Read the model definition and answer for the solid it produces. Units are mm, in the model's axes. Give positions to 0.01 mm unless a question says otherwise; leave off trailing zeros. Loops run counter-clockwise (first coordinate to the right, second up) from the corner with the lowest first, then second, coordinate; pieces in that order, holes last. Notation, with made-up numbers: (86, 4.5) - (130, 4.5) arc R6 cw to (130, 13.5) - close; hole circle Ø11 at (69, 65.25). An arc over 180 degrees is marked (long way). Write each question's results on one line, items separated by ' | '. Start each with the question number.
Q1. Find the intervals of material crossed by line 1 (Y direction, x = -5.5, z = 899); line 2 (Y direction, x = -11.5, z = 1803.4) (3 decimals), in increasing order. Write a range as from..to.
Q2. The part is cut by section B-B, the plane z = 510. Write down the section's boundary in (x, y) (1 decimal).
Q3. The part is cut by section A-A, the plane x = -2. Write down the section's boundary in (y, z), plus the area to 3 significant figures.
```python
from build123d import *

# Parameters (mm, degrees)
SKETCH1_W           = 25.4
SKETCH1_H           = 25.4
SKETCH1_W_2         = 22.225
SKETCH1_H_2         = 22.225
BOSS_EXTRUDE1_DEPTH = 1828.8
SKETCH2_R           = 3.175
CUT_EXTRUDE1_DEPTH  = 26.4
CUT_EXTRUDE2_DEPTH  = 26.4


with BuildPart() as part:
    # Sketch1 → Boss-Extrude1 (new body)
    with BuildSketch(Plane.XY):
        Rectangle(SKETCH1_W, SKETCH1_H)
        Rectangle(SKETCH1_W_2, SKETCH1_H_2, mode=Mode.SUBTRACT)
    extrude(amount=BOSS_EXTRUDE1_DEPTH)

    # Sketch2 → Cut-Extrude1 (cut, through all)
    with BuildSketch(Plane(origin=(12.7, 0, 0), x_dir=(0, 0, -1), z_dir=(1, 0, 0))):
        with Locations((-1727.2, 0)):
            Circle(SKETCH2_R)
        with Locations((-1803.4, 0)):
            Circle(SKETCH2_R)
    extrude(amount=-CUT_EXTRUDE1_DEPTH, mode=Mode.SUBTRACT)

    # Sketch3 → Cut-Extrude2 (cut, through all)
    with BuildSketch(Plane(origin=(12.7, 0, 0), x_dir=(0, 0, -1), z_dir=(1, 0, 0))):
        with BuildLine():
            Line((-1676.4, 3.175), (-50.8, 3.175))
            ThreePointArc((-50.8, 3.175), (-47.625, 0), (-50.8, -3.175))
            Line((-50.8, -3.175), (-1676.4, -3.175))
            ThreePointArc((-1676.4, -3.175), (-1679.575, 0), (-1676.4, 3.175))
        make_face()
    extrude(amount=-CUT_EXTRUDE2_DEPTH, mode=Mode.SUBTRACT)


solid = part.part
```
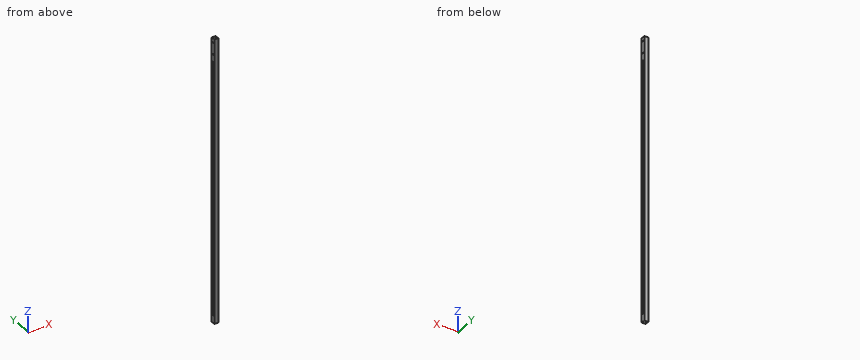
Check sheet entries:
1) line 1: y = -12.7..-11.11, 11.11..12.7 | line 2: y = -12.7..-3.175, 3.175..12.7
2) outline: (-12.7, -12.7) - (12.7, -12.7) - (12.7, -3.2) - (11.1, -3.2) - (11.1, -11.1) - (-11.1, -11.1) - (-11.1, -3.2) - (-12.7, -3.2) - close; (-12.7, 3.2) - (-11.1, 3.2) - (-11.1, 11.1) - (11.1, 11.1) - (11.1, 3.2) - (12.7, 3.2) - (12.7, 12.7) - (-12.7, 12.7) - close
3) outline: (-12.7, 0) - (-11.11, 0) - (-11.11, 1828.8) - (-12.7, 1828.8) - close; (11.11, 0) - (12.7, 0) - (12.7, 1828.8) - (11.11, 1828.8) - close | area: 5,810 mm^2
